Geometry check sheet. Reference: the model listing, model coordinates, mm. Coordinates: 2 decimals unless noted, no trailing zeros. Order: outer loops, then holes, each group sorted by start corner. A loop starts at its lowest first (then second) coordinate and runs counter-clockwise, first axis right, second up. Notation, with made-up numbers: (22, 21) - (69, 21) arc R33 cw to (69, 49) - close; hole circle Ø4 at (19, 88). An arc over 180 degrees is marked (long way). One line per item, written item: value. Start each with the question number.
```python
from build123d import *

# Parameters (mm, degrees)
F0_R     = 10.285065
F0_R_2   = 8.074945
F1_DEPTH = 1.27
F2_R     = 0.508
F3_R     = 0.508
F4_W     = 2.745567
F4_H     = 0.41702
F4_W_2   = 0.434395
F4_H_2   = 0.556026
F5_DEPTH = 0.254


with BuildPart() as f1:
    # F0 (on Front) → F1 (new body, symmetric)
    with BuildSketch(Plane.XZ):
        Circle(F0_R)
        Circle(F0_R_2, mode=Mode.SUBTRACT)
    extrude(amount=F1_DEPTH, both=True)

    # F2
    f2_edges = [f1.edges().sort_by_distance(p)[0] for p in [
        (-10.285065, 1.27, 0),
    ]]
    fillet(f2_edges, radius=F2_R)

    # F3
    f3_edges = [f1.edges().sort_by_distance(p)[0] for p in [
        (-10.285065, -1.27, 0),
    ]]
    fillet(f3_edges, radius=F3_R)

    # F4 (on face) → F5 (cut)
    with BuildSketch(Plane.XZ.offset(1.27)):
        with Locations((1.372783, 8.740652)):
            Rectangle(F4_W, F4_H)
        with Locations((-1.372783, 8.740652)):
            Rectangle(F4_W, F4_H)
        Polygon((0, -8.878413), (0, -9.05217), (1.372878, -9.05217), (1.372878, -8.878413), (0.938483, -8.878413), align=None)
        Polygon((-1.372878, -9.05217), (0, -9.05217), (0, -8.878413), (-0.938483, -8.878413), (-1.372878, -8.878413), align=None)
        with Locations((1.15568, -8.6004)):
            Rectangle(F4_W_2, F4_H_2)
        with Locations((-1.15568, -8.6004)):
            Rectangle(F4_W_2, F4_H_2)
    extrude(amount=-F5_DEPTH, mode=Mode.SUBTRACT)


solid = f1.part
```
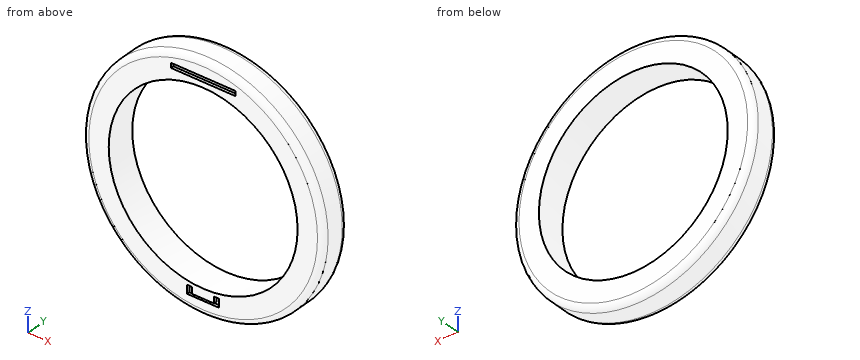
Q1. Cross-section at B-B, the plane z = 0. Enter the section's corners in (x, y), and give its area (3 significant figures).
Q2. Cross-section at C-C, the plane y = 0.15. Enter the section's corners in (x, z).
Q3. Cross-section at A-A, the plane x = 0. Enter the section's corners in (y, z).
Q4. Material ranges on probe 1 along Z at (x, y) = (0, 0.6); probe 2 along Z at (x, y) = (2.25, -1.1); probe 3 along Z at (x, y) = (3.25, -0.8), recorded low to high.
Q5. Gauge pin test, flat end, axial feed: P1, Ø1, axis at x = -2, y = 0, coming from the -Z side. Record the tip position at first contact, or that the pin passes through.
Check result:
1. outline: (-10.29, -0.76) arc R0.51 ccw to (-9.78, -1.27) - (-8.07, -1.27) - (-8.07, 1.27) - (-9.78, 1.27) arc R0.51 ccw to (-10.29, 0.76) - close; (8.07, -1.27) - (9.78, -1.27) arc R0.51 ccw to (10.29, -0.76) - (10.29, 0.76) arc R0.51 ccw to (9.78, 1.27) - (8.07, 1.27) - close
1. area: 11.0 mm2
2. outline: circle Ø20.57 at (0, 0); hole circle Ø16.15 at (0, 0)
3. outline: (-1.27, -9.78) arc R0.51 ccw to (-0.76, -10.29) - (0.76, -10.29) arc R0.51 ccw to (1.27, -9.78) - (1.27, -8.07) - (-1.27, -8.07) - (-1.27, -8.88) - (-1.02, -8.88) - (-1.02, -9.05) - (-1.27, -9.05) - close; (-1.27, 8.07) - (1.27, 8.07) - (1.27, 9.78) arc R0.51 ccw to (0.76, 10.29) - (-0.76, 10.29) arc R0.51 ccw to (-1.27, 9.78) - (-1.27, 8.95) - (-1.02, 8.95) - (-1.02, 8.53) - (-1.27, 8.53) - close
4. probe 1: z = -10.29 to -8.07, 8.07 to 10.29
4. probe 2: z = -9.9 to -7.76, 7.76 to 8.53, 8.95 to 9.9
4. probe 3: z = -9.76 to -7.39, 7.39 to 9.76
5. P1: stops at z = -10.18
